Source: three-view drawing plus pictorial views. Frame: mm from the lowest corner of the part. A direction names the side the tool comes from. Coordinates: 2 decimals unless noted, no trailing zeros. Loops run counter-clockwise (first coordinate to the right, second up) from the corner with the lowest first, then second, coordinate; pieces in that order, holes last. Notation, with made-up numbers: (0.5, 75) - (34.5, 75) arc R37 cw to (34.5, 112) - close; hole circle Ø2 at (86, 69.25). An arc over 180 degrees is marked (long way). Return JSON: item names as keys, results as strings.
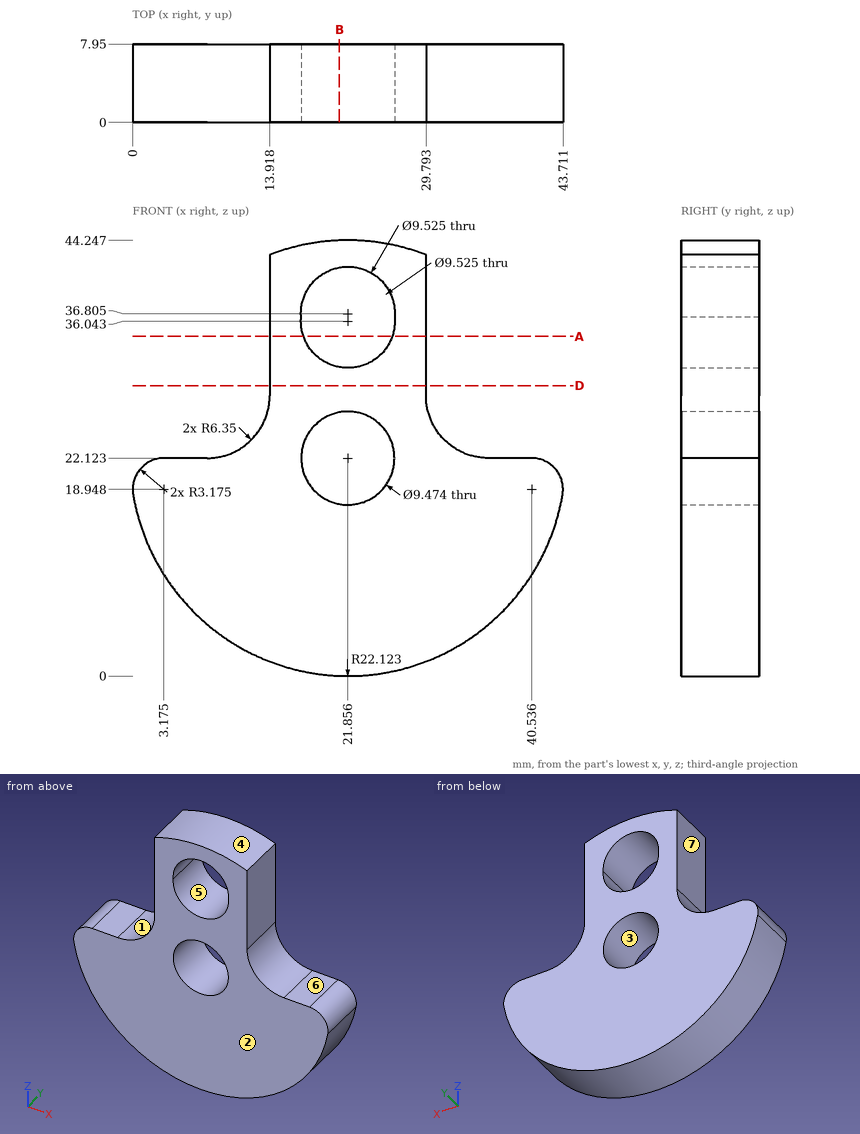
Item 1: Mould query, pull axis Z, two halves, no side actions, for the marked faces 1, 2 and 3. Classes: +Z half, -Z half, draft (parallel to the pull), parting line (faces both ways), or undercut.
Worked out:
{"face 1": "+Z half", "face 2": "draft", "face 3": "undercut"}
Item 2: Reachability of the marked faces 4, 5, 6 and 7 from +Z, -Z, +X, -X, +Y, -Y: full face, straight path, thin tool, end or side. Return the list, or none.
Worked out:
{"face 4": "+Z, +Y, -Y", "face 5": "+Y, -Y", "face 6": "+Z, +X, +Y, -Y", "face 7": "+Z, -X, +Y, -Y"}
Item 3: Ray query, probe 1 along Z at (x, y) = (22, 4) (1 decimal); probe 2 along Z at (x, y) = (24.5, 2.25) (1 decimal); probe 3 along X at (y, z) = (4.75, 37) (1 decimal). Return the intervals inside material, ascending. Write a range as from..to.
Worked out:
{"probe 1": "0..17.4, 26.9..31.3, 41.6..44.2", "probe 2": "0.2..18.2, 26.1..32.1, 40.8..44.1", "probe 3": "13.9..17.1, 26.6..29.8"}
Item 4: Section query A-A, the plane z = 34.5. Return loops of the section in (x, y).
Worked out:
{"outline": "(13.92, 0) - (17.35, 0) - (17.35, 7.95) - (13.92, 7.95) - close; (26.36, 0) - (29.79, 0) - (29.79, 7.95) - (26.36, 7.95) - close"}
Item 5: Section query D-D, the plane z = 29.5. Return loops of the section in (x, y).
Worked out:
{"outline": "(13.92, 0) - (29.79, 0) - (29.79, 7.95) - (13.92, 7.95) - close"}
Item 6: First-contact query: pin 1 Ø7.5 at (x, z) = (21.86, 36.8) entering from +Y; pin 2 Ø15 at (x, z) = (21.86, 22.12) entering from -Y; pin 3 Ø1 at (y, z) = (5, 28) entering from +X; pin 4 Ø3 at (x, y) = (26.5, 4.5) entering from +Z. Flat tips, straight axial feed; report the tip coordinate or a pass-through.
Worked out:
{"pin 1": "through", "pin 2": "y = 0", "pin 3": "x = 29.87", "pin 4": "z = 44.02"}
Item 7: Section query B-B, the plane x = 21. Count the separate pieces of the cut face and the enclosed holes in it, and give its area (3 significant figures).
Worked out:
{"separate pieces": "3", "enclosed holes": "0", "area": "197 mm^2"}
